from build123d import *
from build123d import SkipClean  # not in build123d's __all__

# Parameters (mm, degrees)
F1_DEPTH = 15.875
F4_D     = 6.35
F4_DEPTH = 63.246
F4_TIP   = 1.9077324654
F5_COUNT = 6
F5_ANGLE = 150


with BuildPart() as f1:
    # F0 (on Top) → F1 (new body)
    with BuildSketch(Plane.XY):
        with BuildLine():
            ThreePointArc((25.0633892801, -93.5378422033), (0, -96.8375), (-25.0633892801, -93.5378422033))
            Line((-25.0633892801, -93.5378422033), (-29.9938920893, -111.9387291941))
            ThreePointArc((-29.9938920893, -111.9387291941), (0, -115.8875), (29.9938920893, -111.9387291941))
            Line((29.9938920893, -111.9387291941), (25.0633892801, -93.5378422033))
        make_face()
    extrude(amount=F1_DEPTH)

    # F4
    with Locations(Plane.XZ.offset(115.8875)):
        with Locations((0, 7.9375)):
            Hole(F4_D / 2, depth=F4_DEPTH)
            with Locations((0, 0, -(F4_DEPTH + F4_TIP / 2))):  # 118° drill point
                Cone(0, F4_D / 2, F4_TIP, mode=Mode.SUBTRACT)

    # F5: F1 ×6 about axis
    f5_axis = Axis((0, 0, 0), (0, 0, -1))


with BuildPart() as f1_1:
    add(f1.part, clean=False)
    with SkipClean():  # cleaning this boolean's faces spoils the solid; the shape is the same uncleaned
        for i in range(1, F5_COUNT):
            add(f1.part.rotate(f5_axis, i * F5_ANGLE / (F5_COUNT - 1)), clean=False)


solid = f1_1.part
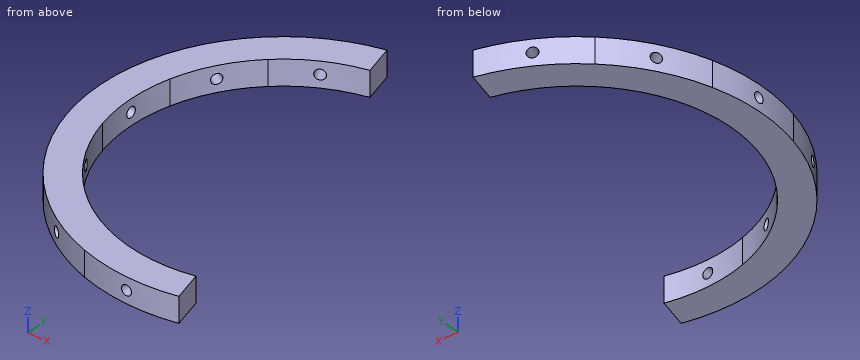
Work out the finished part from the listing and answer in its coordinate system (mm). Give positions to 0.01 mm unless a question says otherwise; leave off trailing zeros. Order: outer loops, then holes, each group sorted by start corner. A loop starts at its lowest first (then second) coordinate and runs counter-clockwise, first axis right, second up. Notation, with made-up numbers: (79, 16.5) -> (110, 16.5) arc R35 cw to (110, 50.5) -> close; hole circle Ø10 at (31.5, 15.25). An arc over 180 degrees is marked (long way). Answer as a JSON object with one key per item and string values. Group by question number.
1. Consider line 1 along Z through (x, y) = (-102.25, 0) (1 decimal); line 2 along Y through (x, z) = (-2, 4); line 3 along Y through (x, z) = (-40, 10.25). Determine where each line is inside the solid, lowest interval first. Write a range as [from, to].
2. Section A-A on y = 0 is taken. Determine the outline of the cut face in (x, z) (1 decimal).
3. Flat-ended cylindrical pins translate along their axes: pin 1 Ø4 at (x, z) = (-61.5, 6) entering from -Y; pin 2 Ø8.5 at (y, z) = (0, 7.94) entering from +X; pin 3 Ø3 at (x, z) = (-15, 2.5) entering from -Y. Find the tip coordinate at first contact, or state that the pin passes through.
4. Section C-C on y = -35.5 is taken. Determine the outline of the cut face in (x, z) (3 decimals), plus the area to 3 significant figures.
Result sheet:
{
 "1": {"line 1": "z = [0, 4.8], [11.1, 15.9]", "line 2": "y = [-115.87, -96.82]", "line 3": "y = [-108.77, -88.19], [88.19, 108.77]"},
 "2": {"outline": "(-115.9, 0) -> (-96.8, 0) -> (-96.8, 4.8) -> (-115.9, 4.8) -> close; (-115.9, 11.1) -> (-96.8, 11.1) -> (-96.8, 15.9) -> (-115.9, 15.9) -> close"},
 "3": {"pin 1": "stops at y = -99.39", "pin 2": "stops at x = -96.74", "pin 3": "stops at y = -115.1"},
 "4": {"outline": "(-110.316, 0) -> (-90.096, 0) -> (-90.096, 15.875) -> (-110.316, 15.875) -> close", "area": "321 mm^2"}
}
